Work out the finished part from the listing and answer in its coordinate system (mm). A direction names the side the tool comes from. Give positions to 0.01 mm unless a question says otherwise; leave off trailing zeros. Loops run counter-clockwise (first coordinate to the right, second up) from the corner with the lowest first, then second, coordinate; pieces in that order, holes last.
```python
from build123d import *

# Parameters (mm, degrees)
SKETCH_1_W            = 32
SKETCH_1_H            = 20
EXTRUDE_1_DEPTH       = 2
SKETCH_2_R            = 3.5
EXTRUDE_2_DEPTH       = 2
HOLE_WIZARD_3_0_3_1_D = 3
SKETCH_5_W            = 2
SKETCH_5_H            = 16
EXTRUDE_3_DEPTH       = 3.8
FILLET_1_DEPTH        = 2
FILLET_START          = -1
FILLET_1_2_DEPTH      = 6.8
FILLET_START_2        = -12
FILLET_1_3_DEPTH      = 24


with BuildPart() as part:
    # 草圖1 → 填料-伸長1 (new body)
    with BuildSketch(Plane.XY):
        Rectangle(SKETCH_1_W, SKETCH_1_H)
    extrude(amount=EXTRUDE_1_DEPTH)

    # 草圖2 → 填料-伸長2 (add)
    with BuildSketch(Plane(origin=(0, 0, 0), x_dir=(-1, 0, 0), z_dir=(0, 0, -1))):
        with Locations((-16, -10)):
            Circle(SKETCH_2_R)
    extrude_2 = extrude(amount=-EXTRUDE_2_DEPTH)

    # Ø3.0 (3) 直徑孔1 (through all)
    with Locations(Plane(origin=(0, 0, 0), x_dir=(-1, 0, 0), z_dir=(0, 0, -1))):
        with Locations((-16, -10)):
            hole_wizard_3_0_3_1 = Hole(HOLE_WIZARD_3_0_3_1_D / 2)

    # 鏡射1: 填料-伸長2, Ø3.0 (3) 直徑孔1 across plane
    add(extrude_2.mirror(Plane(origin=(0, 0, 0), x_dir=(0, 0, 1), z_dir=(1, 0, 0))))
    add(hole_wizard_3_0_3_1.mirror(Plane(origin=(0, 0, 0), x_dir=(0, 0, 1), z_dir=(1, 0, 0))), mode=Mode.SUBTRACT)

    # 草圖5 → 填料-伸長3 (add)
    with BuildSketch(Plane.XY.offset(2)):
        with Locations((-11, 2)):
            Rectangle(SKETCH_5_W, SKETCH_5_H)
    extrude_3 = extrude(amount=EXTRUDE_3_DEPTH)

    # 鏡射2: 填料-伸長3 across plane
    add(extrude_3.mirror(Plane(origin=(0, 0, 0), x_dir=(0, 0, 1), z_dir=(1, 0, 0))))

    # 圓角1: read off the stored shape, not the designer's step
    # 圓角1 outline → 圓角1 (add)
    with BuildSketch(Plane.XY):
        with BuildLine():
            add(Edge.make_bspline(
                [(-17.615384615, -6.895079301), (-16, -6.054649639), (-16, -4.233718703)],
                knots=[0, 0, 0, 1, 1, 1], degree=2, weights=[1, 0.854850414, 1]))
            ThreePointArc((-17.615384615, -6.895079301), (-16.831497912, -6.600204238), (-16, -6.5))
            Line((-16, -6.5), (-16, -4.233718703))
        make_face()
        with BuildLine():
            ThreePointArc((-12.5, -10), (-12.600204238, -10.831497912), (-12.895079301, -11.615384615))
            add(Edge.make_bspline(
                [(-10.233718703, -10), (-12.054649639, -10), (-12.895079301, -11.615384615)],
                knots=[0, 0, 0, 1, 1, 1], degree=2, weights=[1, 0.854850414, 1]))
            Line((-10.233718703, -10), (-12.5, -10))
        make_face()
        with BuildLine():
            Line((12.5, -10), (10.233718703, -10))
            add(Edge.make_bspline(
                [(12.895079301, -11.615384615), (12.054649639, -10), (10.233718703, -10)],
                knots=[0, 0, 0, 1, 1, 1], degree=2, weights=[1, 0.854850414, 1]))
            ThreePointArc((12.895079301, -11.615384615), (12.600204238, -10.831497912), (12.5, -10))
        make_face()
        with BuildLine():
            ThreePointArc((16, -6.5), (16.831497912, -6.600204238), (17.615384615, -6.895079301))
            add(Edge.make_bspline(
                [(16, -4.233718703), (16, -6.054649639), (17.615384615, -6.895079301)],
                knots=[0, 0, 0, 1, 1, 1], degree=2, weights=[1, 0.854850414, 1]))
            Line((16, -4.233718703), (16, -6.5))
        make_face()
    extrude(amount=FILLET_1_DEPTH)

    # Fillet 1 2 outline → Fillet 1 2 (cut)
    with BuildSketch(Plane.XY.offset(FILLET_START)):
        with BuildLine():
            Line((-16, 10), (-16, 7))
            add(Edge.make_bspline(
                [(-16, 7), (-16, 10), (-13, 10)],
                knots=[0, 0, 0, 1, 1, 1], degree=2, weights=[1, 0.707106781, 1]))
            Line((-13, 10), (-16, 10))
        make_face()
        with BuildLine():
            add(Edge.make_bspline(
                [(13, 10), (16, 10), (16, 7)],
                knots=[0, 0, 0, 1, 1, 1], degree=2, weights=[1, 0.707106781, 1]))
            Line((16, 7), (16, 10))
            Line((16, 10), (13, 10))
        make_face()
    extrude(amount=FILLET_1_2_DEPTH, mode=Mode.SUBTRACT)

    # Fillet 1 3 outline → Fillet 1 3 (cut)
    with BuildSketch(Plane.YZ.offset(FILLET_START_2)):
        with BuildLine():
            add(Edge.make_bspline(
                [(10, 2.8), (10, 5.8), (7, 5.8)],
                knots=[0, 0, 0, 1, 1, 1], degree=2, weights=[1, 0.707106781, 1]))
            Line((10, 2.8), (10, 5.8))
            Line((10, 5.8), (7, 5.8))
        make_face()
        with BuildLine():
            add(Edge.make_bspline(
                [(-6, 2.8), (-6, 5.8), (-3, 5.8)],
                knots=[0, 0, 0, 1, 1, 1], degree=2, weights=[1, 0.707106781, 1]))
            Line((-3, 5.8), (-6, 5.8))
            Line((-6, 5.8), (-6, 2.8))
        make_face()
    extrude(amount=FILLET_1_3_DEPTH, mode=Mode.SUBTRACT)


solid = part.part
```
Q1. Which of the six approach directions +Z, -Z, +X, -X, +Y, -Y give full straight-line access (tool end or side, diameter ignored) to faces 1 (the face through (12, 2, 4)), 2 (the face through (10, 2, 4)), 3 (the face through (-16, 1, 1))?
Q2. Section A-A on y = -1 is taken. Give the vertices of the cut face in (x, z).
Q3. Determine the mould class of faces 4 (the face through (0, -10, 1)), 5 (the face through (14.8, -10.9, 1)), 6 (the face through (0, -2, 2)) for opening direction Y: +Y half, -Y half, draft (parallel to the pull), parting line (faces both ways), or undercut.
Q4. Section B-B on x = 2 is taken. Give the vertices of the cut face in (y, z), plus the area to 3 significant figures.
Q5. Consider line 1 along X through (y, z) = (-1.5, 2.65); line 2 along X through (y, z) = (3.75, 1.9); line 3 along Z through (x, y) = (2.5, -4.5). Determine where each line is inside the solid, lowest interval first.
Q6. Given pin 1 (2 mm diameter, centred on x = -14.5, y = -2.5, fed in from +Z); pin 2 (2 mm diameter, centred on x = -2.5, z = 1.5, fed in from -Y); pin 3 (2.5 mm diameter, centred on x = 16, y = -10, fed in from -Z); pin 4 (1.6 mm diameter, centred on y = 3, z = 1, fed in from -X), each flat-ended and moving along its own axis, determine where each tip first touches the part or whether it passes through.
Check result:
1. face 1: +Z, +X, +Y, -Y
1. face 2: +Z, +Y, -Y
1. face 3: +Z, -Z, -X, +Y
2. outline: (-16, 0) - (16, 0) - (16, 2) - (12, 2) - (12, 5.8) - (10, 5.8) - (10, 2) - (-10, 2) - (-10, 5.8) - (-12, 5.8) - (-12, 2) - (-16, 2) - close
3. face 4: -Y half
3. face 5: undercut
3. face 6: draft
4. outline: (-10, 0) - (10, 0) - (10, 2) - (-10, 2) - close
4. area: 40.0 mm2
5. line 1: x = -12 to -10, 10 to 12
5. line 2: x = -16 to 16
5. line 3: z = 0 to 2
6. pin 1: stops at z = 2
6. pin 2: stops at y = -10
6. pin 3: passes through
6. pin 4: stops at x = -16
